For this review, use the dimensioned drawing (mm, ordinates from the lowest corner) and the shaded views. A direction names the side the tool comes from. Coordinates: 2 decimals unless noted, no trailing zeros. Loops run counter-clockwise (first coordinate to the right, second up) from the corner with the lowest first, then second, coordinate; pieces in that order, holes last. Notation, with made-up numbers: M 83.25,49.25 L 142.25,49.25 A36 ccw 142.25,83.25 Z; hole C 24,85 d8. An arc over 180 degrees is marked long. Write item = value, one per line. Start each with the question number.
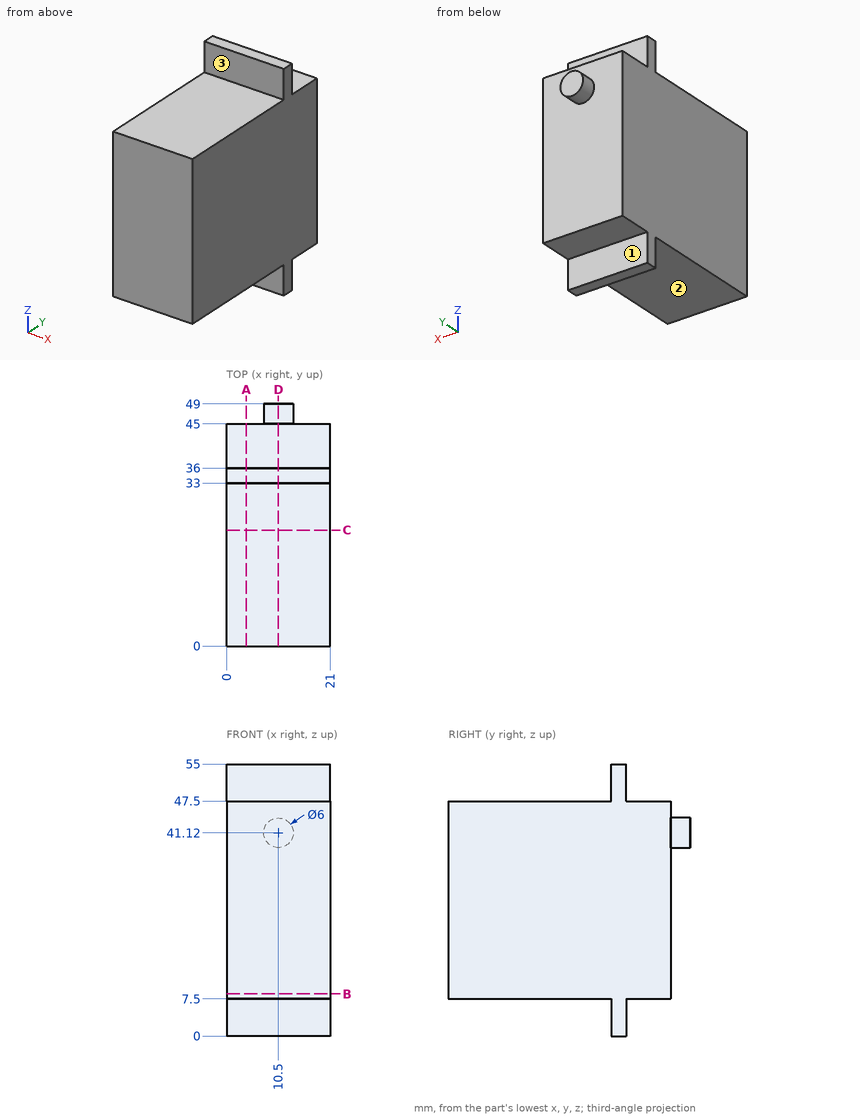
Q1. Add section A-A on x = 4. State the section outline as (y, z) points.
Q2. Add section D-D on x = 10.5. State the section outline as (y, z) points, plus the area to 3 significant figures.
Q3. Add section B-B on z = 8.5. State the section outline as (x, y) points, plus the area to 3 significant figures.
Q4. Add section C-C on y = 23.5. State the section outline as (x, z) points, plus the area to 3 significant figures.
Q5. For the marked faces 1, 2 and 3, list the 3-axis set-ups (+Z, -Z, +X, -X, +Y, -Y) from which the entire face can be reached by the end or side of a thin tool; tool diameter is ignored.
Q6. To check wall thickness, follow line 1 (Z direction, x = 7, y = 23); line 2 (Y direction, x = 9.25, z = 17); line 3 (Y direction, x = 16.5, z = 48.5). State the ranges of each line that lie inside material, in increasing order. Write a range as from..to.
Q7. Clearance check with flat-ended pins moving along their axes: P1, Ø2.5, axis at x = 11, y = 39, coming from the -Z side; P2, Ø2, axis at x = 11.5, y = 31, coming from the +Z side; P3, Ø6, axis at x = 14.5, z = 52.5, coming from the +Y side. State where each tip first meets the part, or that it passes through.
Values follow:
q1.outline = M 0,7.5 L 33,7.5 L 33,0 L 36,0 L 36,7.5 L 45,7.5 L 45,47.5 L 36,47.5 L 36,55 L 33,55 L 33,47.5 L 0,47.5 Z
q2.outline = M 0,7.5 L 33,7.5 L 33,0 L 36,0 L 36,7.5 L 45,7.5 L 45,38.12 L 49,38.12 L 49,44.12 L 45,44.12 L 45,47.5 L 36,47.5 L 36,55 L 33,55 L 33,47.5 L 0,47.5 Z
q2.area = 1,870 mm2
q3.outline = M 0,0 L 21,0 L 21,45 L 0,45 Z
q3.area = 945 mm2
q4.outline = M 0,7.5 L 21,7.5 L 21,47.5 L 0,47.5 Z
q4.area = 840 mm2
q5.face_1 = -Z, +X, -X, +Y
q5.face_2 = -Z, +X, -X, -Y
q5.face_3 = +Z, +X, -X, -Y
q6.line_1 = 7.5..47.5
q6.line_2 = 0..45
q6.line_3 = 33..36
q7.P1 = 7.5
q7.P2 = 47.5
q7.P3 = 36
